For this review, take the finished solid that the model builds, in its own axes (mm). Face numbers are marked on the shaded views. Coordinates: 2 decimals unless noted, no trailing zeros. Write each loop counter-clockwise with the first axis right and the second up, starting at its lowest first coordinate (ties: lowest second). Pieces come first, ordered by that corner, then holes. Notation, with made-up numbers: (-21.75, -18) -> (22.25, -18) arc R33 cw to (22.25, 17) -> close; hole circle Ø4 at (63.25, 12.25). An arc over 180 degrees is marked (long way). Put each result on its own line as item: value. Start each with the question number.
Item 1: To check wall thickness, follow L1, parallel to Z at x = 1, y = -9; L2, parallel to Z at x = 8, y = -7.5; L3, parallel to X at y = 7.5, z = 6. State the ranges of each line that lie inside material, in increasing order.
Item 2: Consider section A-A on y = 0. Give the boundary of the cut face in (x, z), and give its area (3 significant figures).
Item 3: Consider section C-C on z = 3. Give the boundary of the cut face in (x, y).
Item 4: Consider section D-D on z = 43. Give the boundary of the cut face in (x, y).
Item 5: The part is to be moulded in two halves that separate along X. For the marked faces 1 and 2, say which applies: +X half, -X half, draft (parallel to the pull), parting line (faces both ways), or undercut.
Item 6: Insertion check: P1, Ø4, axis at x = -10, y = -1, coming from the -Z side; P2, Ø0.9, axis at x = 7.5, y = 7.5, coming from the -Z side; P3, Ø2, axis at x = 11, z = 41.5, coming from the +Y side. Each pin has a flat end and moves straight along its axis. Give the tip position at first contact, or say it passes through.
```python
from build123d import *

# Parameters (mm, degrees)
F0_R            = 1.5
F1_DEPTH        = 19
F0_R_2          = 6
F2_DEPTH        = 3
F0_R_3          = 15.5
F3_DEPTH        = 66
F4_DEPTH        = 10
F4_COPIES_COUNT = 4


# Not quite as in the source:
# - a pattern or mirror of a feature is missing from the dataset's text; its kind, count and spacing are read off the source's solid


with BuildPart() as f1:
    # F0 (on Top) → F1 (new body)
    with BuildSketch(Plane.XY):
        Circle(F0_R)
    extrude(amount=-F1_DEPTH)

    # F0 (on Top) → F2 (join)
    with BuildSketch(Plane.XY):
        Circle(F0_R_2)
        Circle(F0_R, mode=Mode.SUBTRACT)
    extrude(amount=-F2_DEPTH)

    # F0 (on Top) → F3 (join)
    with BuildSketch(Plane.XY):
        Circle(F0_R_3)
        Circle(F0_R_2, mode=Mode.SUBTRACT)
        with Locations((7.7781745931, 7.7781745931)):
            Circle(F0_R, mode=Mode.SUBTRACT)
        Circle(F0_R_2)
        Circle(F0_R, mode=Mode.SUBTRACT)
        Circle(F0_R)
        with Locations((7.7781745931, 7.7781745931)):
            Circle(F0_R)
    extrude(amount=F3_DEPTH)

    # F0 (on Top) → F4 (cut)
    with BuildSketch(Plane.XY):
        with Locations((7.7781745931, 7.7781745931)):
            Circle(F0_R)
    f4 = extrude(amount=F4_DEPTH, mode=Mode.SUBTRACT)

    # F4_copies: F4 ×4 about axis
    f4_copies_axis = Axis((0, 0, 0), (0, 0, 1))
    for i in range(1, F4_COPIES_COUNT):
        add(f4.rotate(f4_copies_axis, i * 360 / F4_COPIES_COUNT), mode=Mode.SUBTRACT)


solid = f1.part
```
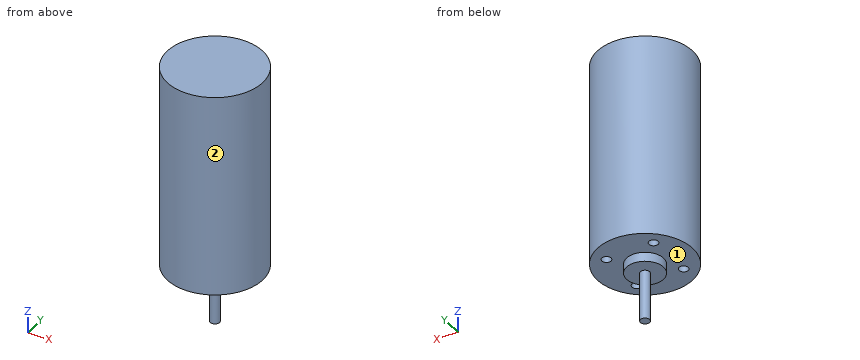
Return value:
1. L1: 0 to 66
1. L2: 10 to 66
1. L3: -13.56 to -9.25, -6.3 to 6.3, 9.25 to 13.56
2. outline: (-15.5, 0) -> (-6, 0) -> (-6, -3) -> (-1.5, -3) -> (-1.5, -19) -> (1.5, -19) -> (1.5, -3) -> (6, -3) -> (6, 0) -> (15.5, 0) -> (15.5, 66) -> (-15.5, 66) -> close
2. area: 2,130 mm^2
3. outline: circle Ø31 at (0, 0); hole circle Ø3 at (-7.78, -7.78); hole circle Ø3 at (-7.78, 7.78); hole circle Ø3 at (7.78, -7.78); hole circle Ø3 at (7.78, 7.78)
4. outline: circle Ø31 at (0, 0)
5. face 1: draft
5. face 2: parting line
6. P1: z = 0
6. P2: z = 10
6. P3: y = 11.84
